The drawing under review shows one solid part. Ordinate dimensions are in mm from its lowest x, y, z. Coordinates: 2 decimals unless noted, no trailing zeros. Write each loop counter-clockwise with the first axis right and the second up, starting at its lowest first coordinate (ties: lowest second). Pieces come first, ordered by that corner, then holes.
Q1. Take a section at A-A (x = 1900). Give the boundary of the cut face in (y, z), and give its area (3 significant figures).
Q2. Mouldability with a two-part tool opening along Y and no side actions: class the marked faces 1 and 2 as pulls with the +Y half, pulls with the -Y half, needs draft (parallel to the pull), parting line crosses it, or undercut.
Q3. For probe 1 along Z at (x, y) = (1084, 627.5); probe 2 along X at (y, z) = (767, 709.5); probe 3 along X at (y, z) = (845.5, 160), list the stretches that pass through material, from the lowest coordinate up.
Q4. Take a section at C-C (y = 100). Give the boundary of the cut face in (x, z), and give its area (3 significant figures).
Q5. Insertion check: pin 1 (12 mm diameter, centred on x = 1385, y = 161.5, fed in from -Z); pin 2 (4 mm diameter, centred on y = 807.5, z = 398.5, fed in from -X). Each pin has a flat end and moves straight along its axis. Give the tip position at first contact, or say it passes through.
Q6. Take a section at D-D (y = 267). Give the boundary of the cut face in (x, z).
Q7. Take a section at B-B (z = 443.5). Give the boundary of the cut face in (x, y).
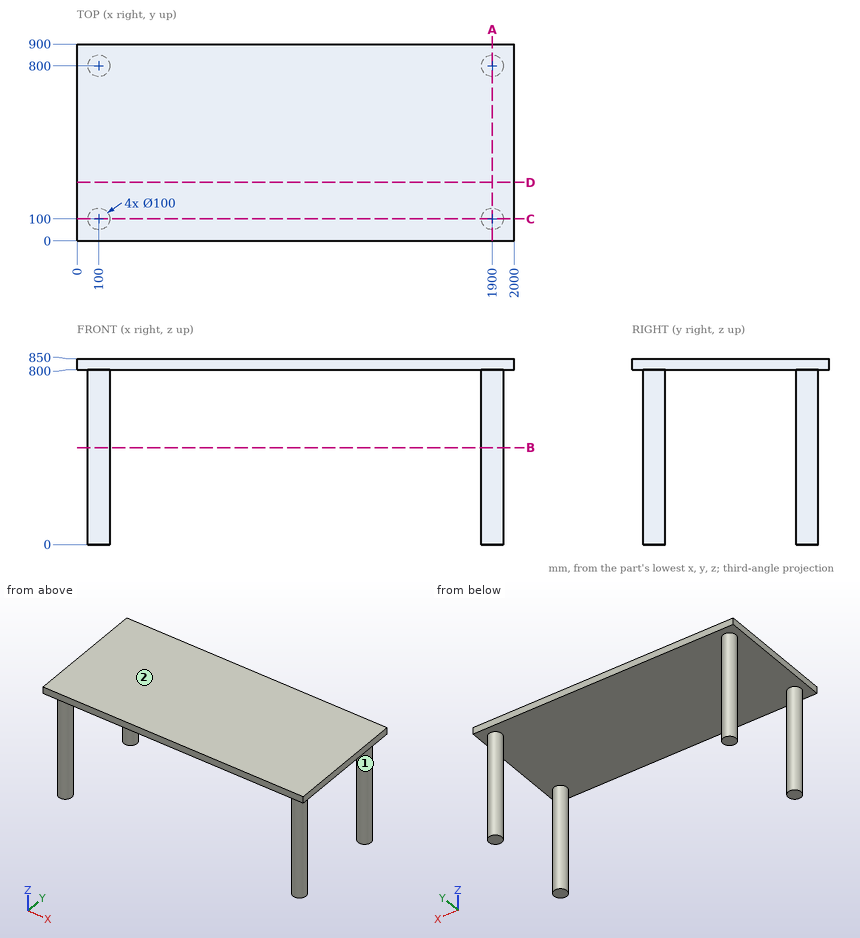
Response:
1. outline: (0, 800) - (50, 800) - (50, 0) - (150, 0) - (150, 800) - (750, 800) - (750, 0) - (850, 0) - (850, 800) - (900, 800) - (900, 850) - (0, 850) - close
1. area: 205,000 mm2
2. face 1: undercut
2. face 2: needs draft
3. probe 1: z = 800 to 850
3. probe 2: x = 62.44 to 137.56, 1862.44 to 1937.56
3. probe 3: x = 79.27 to 120.73, 1879.27 to 1920.73
4. outline: (0, 800) - (50, 800) - (50, 0) - (150, 0) - (150, 800) - (1850, 800) - (1850, 0) - (1950, 0) - (1950, 800) - (2000, 800) - (2000, 850) - (0, 850) - close
4. area: 260,000 mm2
5. pin 1: stops at z = 800
5. pin 2: stops at x = 50.3
6. outline: (0, 800) - (2000, 800) - (2000, 850) - (0, 850) - close
7. outline: circle Ø100 at (100, 100); circle Ø100 at (100, 800); circle Ø100 at (1900, 100); circle Ø100 at (1900, 800)
